Here's how the part is built. I have some questions about the finished solid (model axes, mm). A direction names the side the tool comes from. Round coordinates to 2 decimals unless told otherwise and drop trailing zeros. Order: outer loops, then holes, each group sorted by start corner. A loop starts at its lowest first (then second) coordinate and runs counter-clockwise, first axis right, second up. Notation, with made-up numbers: (7, 64) - (15, 64) arc R30 cw to (15, 103) - close; hole circle Ø3 at (74, 56). An arc over 180 degrees is marked (long way). Answer as a JSON object with one key per item and string values.
```python
from build123d import *

# Parameters (mm, degrees)
SKETCH_1_W          = 41
SKETCH_1_H          = 60
EXTRUDE_1_DEPTH     = 3
SKETCH_2_R          = 1.75
CUT_EXTRUDE_1_DEPTH = 3
FILLET_1_R          = 2
SKETCH_3_W          = 25
SKETCH_3_H          = 8
EXTRUDE_2_DEPTH     = 5
FILLET_2_R          = 1
CHAMFER_2_SIZE      = 1
CHAMFER_1_SIZE      = 2
CUT_EXTRUDE_3_DEPTH = 10


with BuildPart() as part:
    # Эскиз1 → Бобышка-Вытянуть1 (new body)
    with BuildSketch(Plane(origin=(0, 0, 0), x_dir=(1, 0, 0), z_dir=(0, 1, 0))):
        Rectangle(SKETCH_1_W, SKETCH_1_H)
    extrude(amount=EXTRUDE_1_DEPTH)

    # Эскиз2 → Вырез-Вытянуть1 (cut)
    with BuildSketch(Plane(origin=(0, 3, 0), x_dir=(1, 0, 0), z_dir=(0, 1, 0))):
        with Locations(Location((16, 18, 0), (0, 0, 270))):
            Circle(SKETCH_2_R)
        with Locations(Location((16, -18, 0), (0, 0, 90))):
            Circle(SKETCH_2_R)
        with Locations(Location((-16, -18, 0), (0, 0, 270))):
            Circle(SKETCH_2_R)
        with Locations(Location((-16, 18, 0), (0, 0, 90))):
            Circle(SKETCH_2_R)
    extrude(amount=-CUT_EXTRUDE_1_DEPTH, mode=Mode.SUBTRACT)

    # Скругление1
    fillet_1_edges = [part.edges().sort_by_distance(p)[0] for p in [
        (20.5, 1.5, 30),
        (-20.5, 1.5, 30),
        (-20.5, 1.5, -30),
        (20.5, 1.5, -30),
    ]]
    fillet(fillet_1_edges, radius=FILLET_1_R)

    # Эскиз3 → Бобышка-Вытянуть2 (add)
    with BuildSketch(Plane.XZ):
        with Locations((0, 26)):
            Rectangle(SKETCH_3_W, SKETCH_3_H)
    extrude(amount=EXTRUDE_2_DEPTH)

    # Скругление2
    fillet_2_edges = [part.edges().sort_by_distance(p)[0] for p in [
        (12.5, -2.5, 30),
        (-12.5, -2.5, 30),
        (0, -5, 30),
    ]]
    fillet(fillet_2_edges, radius=FILLET_2_R)

    # Фаска2
    chamfer_2_edges = [part.edges().sort_by_distance(p)[0] for p in [
        (0, 3, -30),
        (20.5, 3, 0),
        (-20.5, 3, 0),
        (0, 3, 30),
        (19.914213562, 3, 29.414213562),
        (-19.914213562, 3, 29.414213562),
        (-19.914213562, 3, -29.414213562),
        (19.914213562, 3, -29.414213562),
    ]]
    chamfer(chamfer_2_edges, length=CHAMFER_2_SIZE)

    # Фаска1
    # the kernel refuses this chamfer: 2 mm, written as the material it takes off along each edge
    with BuildSketch(Plane(origin=(-16, 3, -18), x_dir=(0, 0, -1), z_dir=(1, 0, 0))) as chamfer_1_piece_1:
        Polygon((1.75 + CHAMFER_1_SIZE, 0), (1.75, -CHAMFER_1_SIZE), (1.75, 0), align=None)
    revolve(axis=Axis((-16, 3, -18), (0, 1, 0)), mode=Mode.SUBTRACT)
    with BuildSketch(Plane(origin=(-16, 3, 18), x_dir=(0, 0, 1), z_dir=(-1, 0, 0))) as chamfer_1_piece_2:
        Polygon((1.75 + CHAMFER_1_SIZE, 0), (1.75, -CHAMFER_1_SIZE), (1.75, 0), align=None)
    revolve(axis=Axis((-16, 3, 18), (0, 1, 0)), mode=Mode.SUBTRACT)
    with BuildSketch(Plane(origin=(16, 3, 18), x_dir=(0, 0, -1), z_dir=(1, 0, 0))) as chamfer_1_piece_3:
        Polygon((1.75 + CHAMFER_1_SIZE, 0), (1.75, -CHAMFER_1_SIZE), (1.75, 0), align=None)
    revolve(axis=Axis((16, 3, 18), (0, 1, 0)), mode=Mode.SUBTRACT)
    with BuildSketch(Plane(origin=(16, 3, -18), x_dir=(0, 0, 1), z_dir=(-1, 0, 0))) as chamfer_1_piece_4:
        Polygon((1.75 + CHAMFER_1_SIZE, 0), (1.75, -CHAMFER_1_SIZE), (1.75, 0), align=None)
    revolve(axis=Axis((16, 3, -18), (0, 1, 0)), mode=Mode.SUBTRACT)

    # Эскиз4 → Вырез-Вытянуть3 (cut)
    with BuildSketch(Plane(origin=(0, 3, 0), x_dir=(1, 0, 0), z_dir=(0, 1, 0))):
        with BuildLine():
            Line((23.418596888, 22.157492631), (1.187361352, 22.157492631))
            ThreePointArc((1.187361352, 22.157492631), (-6.100332896, 15.822023301), (2.023513442, 10.60169958))
            Line((2.023513442, 10.60169958), (23.418596888, 10.60169958))
            Line((23.418596888, 10.60169958), (23.418596888, 22.157492631))
        make_face()
    extrude(amount=-CUT_EXTRUDE_3_DEPTH, mode=Mode.SUBTRACT)


solid = part.part
```
1. Imagine slicing it at C-C (z = -18). List the corners of the cut face in (x, y) for me (3 decimals).
Responses:
{"outline": "(-20.5, 0) - (-17.75, 0) - (-17.75, 1) - (-19.625, 2.875) - (-20.5, 2) - close; (-14.25, 0) - (-5.859, 0) - (-5.859, 3) - (-12.25, 3) - (-14.25, 1) - close"}
2. Thinking about a two-plate mould opening in Z: for faces 4 (the face through (-6.11, 1.52, -15.98)), 5 (the face through (-20.5, 1, 0)), 6 (the face through (0, 1, -30)), 7 (the face through (11, 2, -10.602)), which applies, pulls with the +Z half, pulls with the -Z half, needs draft (parallel to the pull), parting line crosses it, or undercut?
Responses:
{"face 4": "undercut", "face 5": "needs draft", "face 6": "pulls with the -Z half", "face 7": "undercut"}
3. If I drill on L1, parallel to X at y = 0.7, z = 18; L2, parallel to Z at x = 16, y = 0.85; L3, parallel to Z at x = 8.5, y = 1.25, over which ranges is the centre line in solid material (lowest first)? Write a range as [from, to].
Responses:
{"L1": "[-20.5, -17.75], [-14.25, 14.25], [17.75, 20.5]", "L2": "[-30, -22.16], [-10.6, 16.25], [19.75, 30]", "L3": "[-30, -22.16], [-10.6, 30]"}
4. For P1, Ø6, axis at x = -4, z = -3, coming from the -Y side; P2, Ø4, axis at x = -16, z = -18, coming from the +Y side; P3, Ø2, axis at x = 12, y = -1.5, coming from the -Z side, each with a flat end and sliding along its axis, tell me the tip position at first contact or that it passes through.
Responses:
{"P1": "y = 0", "P2": "y = 1.25", "P3": "z = 22"}
5. Imagine slicing it at B-B (x = -16). List the corners of the cut face in (y, z) for me.
Responses:
{"outline": "(0, -30) - (2, -30) - (3, -29) - (3, -21.75) - (1, -19.75) - (0, -19.75) - close; (0, -16.25) - (1, -16.25) - (3, -14.25) - (3, 14.25) - (1, 16.25) - (0, 16.25) - close; (0, 19.75) - (1, 19.75) - (3, 21.75) - (3, 29) - (2, 30) - (0, 30) - close"}
6. Imagine slicing it at A-A (x = 4). List the corners of the cut face in (y, z) for me.
Responses:
{"outline": "(-5, 22) - (0, 22) - (0, -10.6) - (3, -10.6) - (3, 29) - (2, 30) - (-4, 30) arc R1 ccw to (-5, 29) - close; (0, -30) - (2, -30) - (3, -29) - (3, -22.16) - (0, -22.16) - close"}
7. For faces 1 (the face through (-19.93, 1.01, -29.4)), 2 (the face through (12.5, -2, 25)), 3 (the face through (-12.5, -2, 25)), which set-ups out of +Z, -Z, +X, -X, +Y, -Y let a thin tool reach every point of the face, with its end or its side?
Responses:
{"face 1": "-Z, -X, +Y, -Y", "face 2": "+Z, -Z, +X, -Y", "face 3": "+Z, -Z, -X, -Y"}
8. Imagine slicing it at D-D (y = -2.5). List the corners of the cut face in (x, z) for me.
Responses:
{"outline": "(-12.5, 22) - (12.5, 22) - (12.5, 29) arc R1 ccw to (11.5, 30) - (-11.5, 30) arc R1 ccw to (-12.5, 29) - close"}
